Here's how the part is built. I have some questions about the finished solid (model axes, mm). Face numbers are marked on the shaded views. A direction names the side the tool comes from. Coordinates: 2 decimals unless noted, no trailing zeros. Write each loop counter-clockwise with the first axis right and the second up, starting at its lowest first coordinate (ties: lowest second). Pieces come first, ordered by that corner, then holes. Notation, with made-up numbers: (70, 19.5) - (94, 19.5) arc R20 cw to (94, 50.5) - close; hole circle Ø3 at (23.5, -20). An arc over 180 degrees is marked (long way). Answer in a Markdown table with one row per item. Add a question column.
Item 1: Which directions (+Z, -Z, +X, -X, +Y, -Y) give clear straight access to the entire face, cutting with the end or side of a thin tool? Please do the marked faces 1, 2 and 3.
Item 2: Imagine slicing it at B-B (z = 7.5). Please give me the cut outline in (x, y) (3 decimals), plus the area to 3 significant figures.
Item 3: If I drill on probe 1 along X at (y, z) = (-0.8, 8); probe 2 along X at (y, z) = (-2.4, 8); probe 3 along Y at (x, z) = (55, -15.5) (3 decimals), over which ranges is the centre line in solid material (lowest first)? Write a range as from..to.
Item 4: I'm going to push flat-ended pins straight in: pin 1 (10 mm diameter, centred on x = 48, z = -8, fed in from +Y); pin 2 (5 mm diameter, centred on y = -6.5, z = -2.5, fed in from +X) (3 decimals); pin 3 (3 mm diameter, centred on x = 10, y = -6, fed in from +Z); pin 4 (5.5 mm diameter, centred on y = -7.5, z = -5, fed in from -X). Where does each tip first touch, or does it pass through?
Item 5: Imagine slicing it at D-D (y = -9). Please give me the cut outline in (x, z) (3 decimals).
Item 6: Imagine slicing it at C-C (z = -1). Please give me the cut outline in (x, y) (3 decimals), plus the area to 3 significant figures.
Item 7: Imagine slicing it at A-A (x = 17.5). Please give me the cut outline in (y, z) (3 decimals).
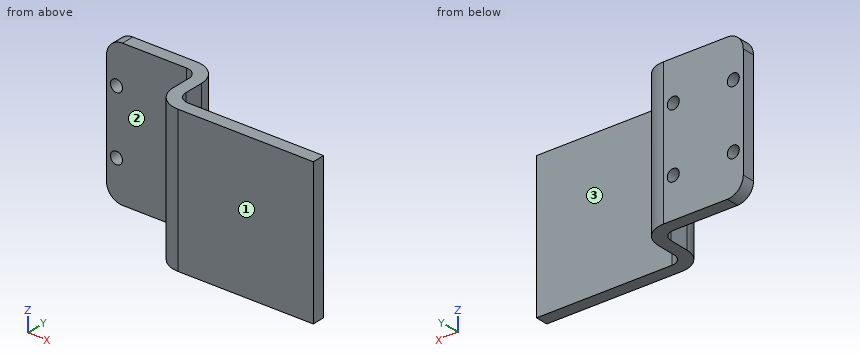
from build123d import *

# Parameters (mm, degrees)
SKETCH2_W                    = 23
SKETCH2_H                    = 36
BASE_FLANGE1_DEPTH           = 3.175
EDGE_FLANGE4_STRIP_W         = 18.7
EDGE_FLANGE4_STRIP_H         = 3.175
EDGE_FLANGE4_STRIP_CUT_DEPTH = 36
EDGE_FLANGE4_DEPTH           = 36
EDGE_FLANGE5_STRIP_W         = 18.7
EDGE_FLANGE5_STRIP_H         = 3.175
EDGE_FLANGE5_STRIP_CUT_DEPTH = 36
EDGE_FLANGE5_DEPTH           = 36
SKETCH20_R                   = 1.5
CUT_EXTRUDE1_DEPTH           = 68.734633866
FILLET1_R                    = 4


# Sheet-metal steps are written as plain solids
with BuildPart() as part:
    # Sketch2 → Base-Flange1 (new body)
    with BuildSketch(Plane(origin=(0, 0, 0), x_dir=(1, 0, 0), z_dir=(0, 1, 0))):
        with Locations((11.5, 0)):
            Rectangle(SKETCH2_W, SKETCH2_H)
    extrude(amount=-BASE_FLANGE1_DEPTH)

    # Edge-Flange4 strip (across the edge) → Edge-Flange4 strip cut (cut)
    with BuildSketch(Plane(origin=(23, -3.175, -18), x_dir=(-1, 0, 0), z_dir=(0, 0, 1))):
        with Locations((-6.35, -1.5875)):
            Rectangle(EDGE_FLANGE4_STRIP_W, EDGE_FLANGE4_STRIP_H)
    extrude(amount=EDGE_FLANGE4_STRIP_CUT_DEPTH, mode=Mode.SUBTRACT)

    # Edge-Flange4 section (across the edge) → Edge-Flange4 (add)
    with BuildSketch(Plane(origin=(23, -3.175, -18), x_dir=(-1, 0, 0), z_dir=(0, 0, 1))):
        with BuildLine():
            Line((-3.175, 3), (-3.175, 10.825))
            Line((-3.175, 10.825), (0, 10.825))
            Line((0, 10.825), (0, 3))
            ThreePointArc((0, 3), (0.878679656, 0.878679656), (3, 0))
            Line((3, 0), (3, -3.175))
            ThreePointArc((3, -3.175), (-1.366384374, -1.366384374), (-3.175, 3))
        make_face()
    extrude(amount=EDGE_FLANGE4_DEPTH)

    # Edge-Flange5 strip (across the edge) → Edge-Flange5 strip cut (cut)
    with BuildSketch(Plane(origin=(26.175, -14, 18), x_dir=(0, 1, 0), z_dir=(0, 0, -1))):
        with Locations((-6.35, -1.5875)):
            Rectangle(EDGE_FLANGE5_STRIP_W, EDGE_FLANGE5_STRIP_H)
    extrude(amount=EDGE_FLANGE5_STRIP_CUT_DEPTH, mode=Mode.SUBTRACT)

    # Edge-Flange5 section (across the edge) → Edge-Flange5 (add)
    with BuildSketch(Plane(origin=(26.175, -14, 18), x_dir=(0, 1, 0), z_dir=(0, 0, -1))):
        with BuildLine():
            Line((-3.175, 3), (-3.175, 36.825))
            Line((-3.175, 36.825), (0, 36.825))
            Line((0, 36.825), (0, 3))
            ThreePointArc((0, 3), (0.878679656, 0.878679656), (3, 0))
            Line((3, 0), (3, -3.175))
            ThreePointArc((3, -3.175), (-1.366384374, -1.366384374), (-3.175, 3))
        make_face()
    extrude(amount=EDGE_FLANGE5_DEPTH)

    # Sketch20 → Cut-Extrude1 (cut, through all)
    with BuildSketch(Plane(origin=(0, 0, 0), x_dir=(1, 0, 0), z_dir=(0, 1, 0))):
        with Locations(Location((17.5, -8, 0), (0, 0, 270))):
            Circle(SKETCH20_R)
        with Locations(Location((17.5, 8, 0), (0, 0, 270))):
            Circle(SKETCH20_R)
        with Locations(Location((2.5, 8, 0), (0, 0, 270))):
            Circle(SKETCH20_R)
        with Locations(Location((2.5, -8, 0), (0, 0, 270))):
            Circle(SKETCH20_R)
    extrude(amount=-CUT_EXTRUDE1_DEPTH, mode=Mode.SUBTRACT)

    # Fillet1
    fillet1_edges = [part.edges().sort_by_distance(p)[0] for p in [
        (0, -1.5875, 18),
        (0, -1.5875, -18),
    ]]
    fillet(fillet1_edges, radius=FILLET1_R)


solid = part.part
Here are the results:
| question | item | result |
|---|---|---|
| 1 | face 1 | +Z, -Z, +X, -X, -Y |
| 1 | face 2 | +Z, -Z, -X, -Y |
| 1 | face 3 | +Z, -Z, +X, +Y |
| 2 | outline | (0, -3.175) - (1.086, -3.175) - (1.086, 0) - (0, 0) - close; (3.914, -3.175) - (16.086, -3.175) - (16.086, 0) - (3.914, 0) - close; (18.914, -3.175) - (20, -3.175) arc R3 cw to (23, -6.175) - (23, -11) arc R6.175 ccw to (29.175, -17.175) - (63, -17.175) - (63, -14) - (29.175, -14) arc R3 cw to (26.175, -11) - (26.175, -6.175) arc R6.175 ccw to (20, 0) - (18.914, 0) - close |
| 2 | area | 214 mm2 |
| 3 | probe 1 | x = 0..1, 4..16, 19..23.04 |
| 3 | probe 2 | x = 0..1, 4..16, 19..24.89 |
| 3 | probe 3 | y = -17.175..-14 |
| 4 | pin 1 | stops at y = -14 |
| 4 | pin 2 | stops at x = 26.175 |
| 4 | pin 3 | passes through |
| 4 | pin 4 | stops at x = 22.64 |
| 5 | outline | (23, -18) - (26.175, -18) - (26.175, 18) - (23, 18) - close |
| 6 | outline | (0, -3.175) - (20, -3.175) arc R3 cw to (23, -6.175) - (23, -11) arc R6.175 ccw to (29.175, -17.175) - (63, -17.175) - (63, -14) - (29.175, -14) arc R3 cw to (26.175, -11) - (26.175, -6.175) arc R6.175 ccw to (20, 0) - (0, 0) - close |
| 6 | area | 232 mm2 |
| 7 | outline | (-3.175, -18) - (0, -18) - (0, -9.5) - (-3.175, -9.5) - close; (-3.175, -6.5) - (0, -6.5) - (0, 6.5) - (-3.175, 6.5) - close; (-3.175, 9.5) - (0, 9.5) - (0, 18) - (-3.175, 18) - close |
